CAD build for the part. Positions are in the model's coordinates, mm. Face numbers are marked on the shaded views. Give positions to 0.01 mm unless a question says otherwise; leave off trailing zeros. Order: outer loops, then holes, each group sorted by start corner. A loop starts at its lowest first (then second) coordinate and runs counter-clockwise, first axis right, second up.
Item 1: Flat gauge pins, fed straight in: P1, Ø5, axis at x = 0, y = 10, coming from the -Z side; P2, Ø6.5, axis at x = -46, y = 10, coming from the +Z side; P3, Ø3, axis at x = 2, y = 1, coming from the -Z side. Where does each tip first touch, or does it go through?
Item 2: Two-plate mould, pull along Y, no slides. Class the marked faces 1, 2 and 3: released by +Y, released by -Y, zero draft, split by the parting line, or undercut.
Item 3: Band-saw the part on D-D on x = 13.5. Give the cut face in (y, z) (3 decimals), plus the area to 4 significant figures.
Item 4: Band-saw the part on B-B on y = 10. Count the separate pieces of the cut face and the enclosed holes in it, plus the area to 3 significant figures.
Item 5: Band-saw the part on A-A on x = -46. Give the cut face in (y, z), plus the area to 3 significant figures.
Item 6: Wall check: L1, parallel to Y at x = -46.5, z = 8.5; L2, parallel to Y at x = -46, z = 2.95; L3, parallel to X at y = -10, z = 2.2. Give the ranges that are in metal, low to high.
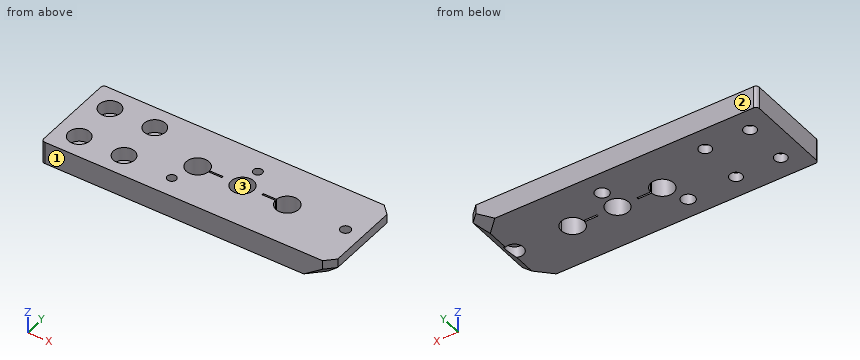
Autodesk Inventor part; units mm, degrees
ref_plane "YZ Plane" through (0, 0, 0) normal (1, 0, 0) x (0, 1, 0)
ref_plane "XZ Plane" through (0, 0, 0) normal (0, 1, 0) x (-1, 0, 0)
ref_plane "XY Plane" through (0, 0, 0) normal (0, 0, 1) x (1, 0, 0)
sketch "Sketch1" plane through (0, 0, 0) normal (0, 0, 1) x (1, 0, 0)
  line L0 (49.5, 20) -> (-74.5, 20)
  line L1 (-76, 18.5) -> (-76, -18.5)
  line L2 (-74.5, -20) -> (49.5, -20)
  line L3 (-102.2728, 0) -> (79.4621, 0) construction
  line L4 (0, 28.4349) -> (0, -28.4349) construction
  circle A0 centre (0, 0) radius 5
  circle A1 centre (20, 0) radius 5.075
  line L5 (14.9389, 0.375) -> (8.9389, 0.375)
  line L6 (8.9389, 0.375) -> (8.9389, 0)
  line L7 (14.9389, -0.375) -> (8.9389, -0.375)
  line L8 (8.9389, -0.375) -> (8.9389, 0)
  circle A2 centre (-20, 0) radius 5.075
  line L9 (-14.9389, 0.375) -> (-8.9389, 0.375)
  line L10 (-8.9389, 0.375) -> (-8.9389, 0)
  line L11 (-14.9389, -0.375) -> (-8.9389, -0.375)
  line L12 (-8.9389, -0.375) -> (-8.9389, 0)
  circle A3 centre (0, 10) radius 2
  line L13 (36, 20) -> (36, -20) construction
  circle A4 centre (-24, -11) radius 2
  circle A5 centre (46, 0) radius 2.25
  line L14 (-46, -10) -> (-66, -10) construction
  line L15 (-66, -10) -> (-66, 10) construction
  line L16 (-66, 10) -> (-46, 10) construction
  line L17 (-46, 10) -> (-46, -10) construction
  line L18 (-46, -10) -> (-66, 10) construction
  line L19 (-66, -10) -> (-46, 10) construction
  circle A6 centre (-66, 10) radius 2.75
  circle A7 centre (-46, 10) radius 2.75
  circle A8 centre (-46, -10) radius 2.75
  circle A9 centre (-66, -10) radius 2.75
  line L20 (0, 15) -> (-45, 15) construction
  line L21 (-45, 15) -> (-45, 0) construction
  line L22 (-45, 0) -> (-30, -15) construction
  line L23 (-30, -15) -> (0, -15) construction
  line L24 (-36, -20) -> (-76, -20) construction
  line L25 (-76, -20) -> (-76, 20) construction
  line L26 (-76, 20) -> (-36, 20) construction
  line L27 (-36, 20) -> (-36, -20) construction
  line L28 (-36, -20) -> (-76, 20) construction
  line L29 (-76, -20) -> (-36, 20) construction
  arc A10 (-76, -18.5) -> (-74.5, -20) centre (-74.5, -18.5) ccw
  arc A11 (-74.5, 20) -> (-76, 18.5) centre (-74.5, 18.5) ccw
  line L30 (53.5, -16) -> (53.5, 16)
  line L31 (53.5, -16) -> (49.5, -20)
  line L32 (49.5, 20) -> (53.5, 16)
  point P0 (0, 0)
  point P1 (-56, 0)
  point P2 (53.5, -20)
  point P3 (53.5, 20)
  point P4 (-14.9389, -0.375)
  point P5 (14.9389, -0.375)
  dimension "d99" = 10.15
  dimension "d44" = 10
  dimension "d46" = 0.75
  dimension "d47" = 6
  dimension "d48" = 40
  dimension "d49" = 4
  dimension "d50" = 10
  dimension "d51" = 16
  dimension "d55" = 11
  dimension "d56" = 4
  dimension "d60" = 10
  dimension "d62" = 20
  dimension "d63" = 10
  dimension "d64" = 5.5
  dimension "d65" = 45
  dimension "d66" = 30
  dimension "d67" = 45
  dimension "d68" = 40
  dimension "d69" = 40
  dimension "d70" = 1.5
  dimension "d73" = 16
  dimension "d86" = 17.5
  dimension "d87" = 40
  dimension "d89" = 4.5
  dimension "d90" = 4
  dimension "d91" = 4
  dimension "d92" = 4
  dimension "d93" = 4
extrude "Vysunutí1" add sketch "Sketch1" along normal blind 10
sketch "Sketch2" plane through (0, 0, 0) normal (0, 0, -1) x (-1, 0, 0)
  circle A0 centre (-46, 0) radius 2.25 construction
  circle A1 centre (-46, 0) radius 2.25
  circle A2 centre (-46, 0) radius 4
  circle A3 centre (0, 10) radius 2 construction
  circle A4 centre (24, -11) radius 2 construction
  circle A5 centre (0, 10) radius 3
  circle A6 centre (24, -11) radius 3
  point P0 (0, 0)
  point P1 (-66, 0)
  dimension "d85" = 6
extrude "Extrusion2" cut sketch "Sketch2" against normal blind 5 contours A1 | A2 | A5 | A6
sketch "Sketch3" plane through (0, 0, 10) normal (0, 0, 1) x (1, 0, 0)
  circle A0 centre (-46, -10) radius 2.75 construction
  circle A1 centre (-66, -10) radius 2.75 construction
  circle A2 centre (-66, 10) radius 2.75 construction
  circle A3 centre (-46, 10) radius 2.75 construction
  circle A4 centre (-46, -10) radius 2.75 construction
  circle A5 centre (-46, -10) radius 4.75
  circle A6 centre (-66, -10) radius 4.75
  circle A7 centre (-66, 10) radius 4.75
  circle A8 centre (-46, 10) radius 4.75
  point P0 (0, 0)
  dimension "d82" = 9.5
extrude "Extrusion3" cut sketch "Sketch3" against normal blind 6
chamfer "Chamfer1" distance 6 angle 45 3 edges at (53.5, 0, 0) (51.5, -18, 0) (51.5, 18, 0)
properties part number "_3DPrint"
The answers:
1. P1: stops at z = 5
1. P2: stops at z = 4
1. P3: passes through
2. face 1: released by -Y
2. face 2: released by +Y
2. face 3: undercut
3. outline: (-20, 0) - (-0.375, 0) - (-0.375, 10) - (-20, 10) - close; (0.375, 0) - (20, 0) - (20, 10) - (0.375, 10) - close
3. area: 392.5 mm2
4. separate pieces: 4
4. enclosed holes: 0
4. area: 1,070 mm2
5. outline: (-20, 0) - (-12.75, 0) - (-12.75, 4) - (-14.75, 4) - (-14.75, 10) - (-20, 10) - close; (-7.25, 0) - (7.25, 0) - (7.25, 4) - (5.25, 4) - (5.25, 10) - (-5.25, 10) - (-5.25, 4) - (-7.25, 4) - close; (12.75, 0) - (20, 0) - (20, 10) - (14.75, 10) - (14.75, 4) - (12.75, 4) - close
5. area: 242 mm2
6. L1: y = -20 to -14.72, -5.28 to 5.28, 14.72 to 20
6. L2: y = -20 to -12.75, -7.25 to 7.25, 12.75 to 20
6. L3: x = -76 to -68.75, -63.25 to -48.75, -43.25 to -26.83, -21.17 to 49.7
